Verification items for the finished model (mm, model axes). A direction names the side the tool comes from. Round coordinates to 2 decimals unless told otherwise and drop trailing zeros. Order: outer loops, then holes, each group sorted by start corner. A loop starts at its lowest first (then second) coordinate and runs counter-clockwise, first axis right, second up. Notation, with made-up numbers: M 21.25,42.25 L 63.25,42.25 A23 cw 63.25,60.25 Z; hole C 77,12.5 d4. An arc over 180 degrees is marked long. Answer as a JSON object with one key per item and string values. Group by question number.
```python
from build123d import *

# Parameters (mm, degrees)
F1_DEPTH = 25.4
F2_DEPTH = 25.4


with BuildPart() as f1:
    # F0 (on Top) → F1 (new body)
    with BuildSketch(Plane.XY):
        Polygon((-29.327272, 32.004528), (-40.825695, 32.004528), (-40.825695, 0), (38.318675, 0), (38.318675, 32.004528), (18.865567, 32.004528), (7.069093, 32.004528), (0, 32.004528), (0, 18.464023), (5.171617, 18.464023), (4.928618, 13.130507), (0, 13.130507), (0, 7.304969), (-8.66149, 7.304969), (-8.66149, 13.279019), (-13.442378, 13.279019), (-13.442378, 18.870654), (-8.66149, 18.870654), (-8.66149, 32.004528), (-17.973778, 32.004528), align=None)
    extrude(amount=F1_DEPTH)

    # F0 (on Top) → F2 (join)
    with BuildSketch(Plane.XY):
        Polygon((-29.327272, 32.004528), (-40.825695, 32.004528), (-40.825695, 0), (38.318675, 0), (38.318675, 32.004528), (18.865567, 32.004528), (7.069093, 32.004528), (0, 32.004528), (0, 18.464023), (5.171617, 18.464023), (4.928618, 13.130507), (0, 13.130507), (0, 7.304969), (-8.66149, 7.304969), (-8.66149, 13.279019), (-13.442378, 13.279019), (-13.442378, 18.870654), (-8.66149, 18.870654), (-8.66149, 32.004528), (-17.973778, 32.004528), align=None)
        Polygon((-29.327272, 42.033378), (-29.327272, 32.004528), (-17.973778, 32.004528), (-18.074421, 42.22302), align=None)
        Polygon((0, 32.004528), (-8.66149, 32.004528), (-8.66149, 18.870654), (-13.442378, 18.870654), (-13.442378, 13.279019), (-8.66149, 13.279019), (-8.66149, 7.304969), (0, 7.304969), (0, 13.130507), (4.928618, 13.130507), (5.171617, 18.464023), (0, 18.464023), align=None)
        Polygon((7.069093, 32.004528), (18.865567, 32.004528), (18.865567, 42.118017), (7.069093, 41.962616), align=None)
    extrude(amount=F2_DEPTH)


solid = f1.part
```
Q1. Gauge pin test, flat ends, axial feed: pin 1 Ø1 at (x, y) = (-4.5, 33) entering from -Z; pin 2 Ø12.5 at (x, z) = (-32.5, 15) entering from +Y; pin 3 Ø5 at (y, z) = (37, 11) entering from -X; pin 4 Ø12.5 at (x, z) = (-7, 18) entering from +Y. Record the tip position at first contact, or that the pin passes through.
Q2. Cross-section at B-B, the plane z = 3.75. Record the cut outline in (x, y), then the cut area to 3 significant figures.
Q3. Release check for a two-part mould opening along X. For faces 1 (the face through (-2, 17, 25.4)), 2 (the face through (-40.826, 16, 13)), 3 (the face through (-5, 32.005, 13)) record: released by +X, released by -X, zero draft, split by the parting line, or undercut.
Q4. Tool access check on faces 4 (the face through (7.069, 37, 13)), 5 (the face through (29, 32.005, 13)), 6 (the face through (-29.327, 37, 13)). Record the directions out of +Z, -Z, +X, -X, +Y, -Y that give a thin tool (end or side, any length) a straight path to the whole face; none if there is none.
Q5. Thickness scan on line 1 (X direction, y = 40.5, z = 14.75); line 2 (Y direction, x = 34.5, z = 4.25); line 3 (Y direction, x = 11, z = 24). Record the ranges inside material, lowest first. Write a range as from..to.
Q6. Cross-section at A-A, the plane y = 39.5. Record the cut outline in (x, z), then the cut area to 3 significant figures.
Q7. Cross-section at C-C, the plane x = -1.5. Record the cut outline in (y, z), then the cut area to 3 significant figures.
Conclusion:
{
 "1": {"pin 1": "through", "pin 2": "y = 42.09", "pin 3": "x = -29.33", "pin 4": "y = 32"},
 "2": {"outline": "M -40.83,0 L 38.32,0 L 38.32,32 L 18.87,32 L 18.87,42.12 L 7.07,41.96 L 7.07,32 L -17.97,32 L -18.07,42.22 L -29.33,42.03 L -29.33,32 L -40.83,32 Z", "area": "2,770 mm2"},
 "3": {"face 1": "zero draft", "face 2": "released by -X", "face 3": "undercut"},
 "4": {"face 4": "+Z, -Z, +Y", "face 5": "+Z, -Z, +X, +Y", "face 6": "+Z, -Z, -X, +Y"},
 "5": {"line 1": "-29.33..-18.06, 7.07..18.87", "line 2": "0..32", "line 3": "0..42.01"},
 "6": {"outline": "M -29.33,0 L -18.05,0 L -18.05,25.4 L -29.33,25.4 Z; M 7.07,0 L 18.87,0 L 18.87,25.4 L 7.07,25.4 Z", "area": "586 mm2"},
 "7": {"outline": "M 0,0 L 32,0 L 32,25.4 L 0,25.4 Z", "area": "813 mm2"}
}
